Check sheet for the modelled part. Datum: model origin and axes. Units: mm. Face numbers are marked on the shaded views. A direction names the side the tool comes from. Coordinates: 2 decimals unless noted, no trailing zeros. Write each loop counter-clockwise with the first axis right and the second up, starting at its lowest first coordinate (ties: lowest second). Pieces come first, ordered by that corner, then holes. Notation, with made-up numbers: (56, 62) -> (87, 62) arc R21 cw to (87, 71) -> close; hole circle Ø10 at (-21.75, 0.5). An arc over 180 degrees is marked (long way). Put each result on its own line as item: value.
```python
from build123d import *

# Parameters (mm, degrees)
SKETCH1_W           = 8
SKETCH1_H           = 3.056305014
BOSS_EXTRUDE1_DEPTH = 1.5


with BuildPart() as part:
    # Sketch1 → Boss-Extrude1 (new, symmetric)
    with BuildSketch(Plane.XY):
        with BuildLine():
            Line((-10.083709216, 9.599779274), (-10.083709216, 6.299779274))
            Line((-10.083709216, 6.299779274), (-12.68296021, 6.299779274))
            ThreePointArc((-12.68296021, 6.299779274), (-13.0365136, 6.153332664), (-13.18296021, 5.799779274))
            Line((-13.18296021, 5.799779274), (-13.18296021, 4.602368782))
            ThreePointArc((-13.18296021, 4.602368782), (-13.376633784, 4.010897992), (-13.882635601, 3.648531727))
            ThreePointArc((-13.882635601, 3.648531727), (-14.651645992, 3.099880506), (-14.950395595, 2.20369759))
            ThreePointArc((-14.950395595, 2.20369759), (-14.575936583, 1.043545253), (-13.583709216, 0.335267166))
            Line((-13.583709216, 0.335267166), (-13.583709216, 1.664695612))
            Line((-13.583709216, 1.664695612), (-10.083709216, 1.664695612))
            Line((-10.083709216, 1.664695612), (-10.083709216, 0.256084288))
            Line((-10.083709216, 0.256084288), (13.916290784, 0.256084288))
            Line((13.916290784, 0.256084288), (13.916290784, 1.664695612))
            Line((13.916290784, 1.664695612), (17.416290784, 1.664695612))
            Line((17.416290784, 1.664695612), (17.416290784, 0.335267166))
            ThreePointArc((17.416290784, 0.335267166), (18.408518152, 1.043545253), (18.782977164, 2.20369759))
            ThreePointArc((18.782977164, 2.20369759), (18.484227561, 3.099880506), (17.715217169, 3.648531727))
            ThreePointArc((17.715217169, 3.648531727), (17.209215353, 4.010897992), (17.015541778, 4.602368782))
            Line((17.015541778, 4.602368782), (17.015541778, 5.799779274))
            ThreePointArc((17.015541778, 5.799779274), (16.869095169, 6.153332664), (16.515541778, 6.299779274))
            Line((16.515541778, 6.299779274), (13.916290784, 6.299779274))
            Line((13.916290784, 6.299779274), (13.916290784, 9.599779274))
            Line((13.916290784, 9.599779274), (-10.083709216, 9.599779274))
        make_face()
        with Locations((1.916290784, 4.927931781)):
            Rectangle(SKETCH1_W, SKETCH1_H, mode=Mode.SUBTRACT)
    extrude(amount=BOSS_EXTRUDE1_DEPTH, both=True)


solid = part.part
```
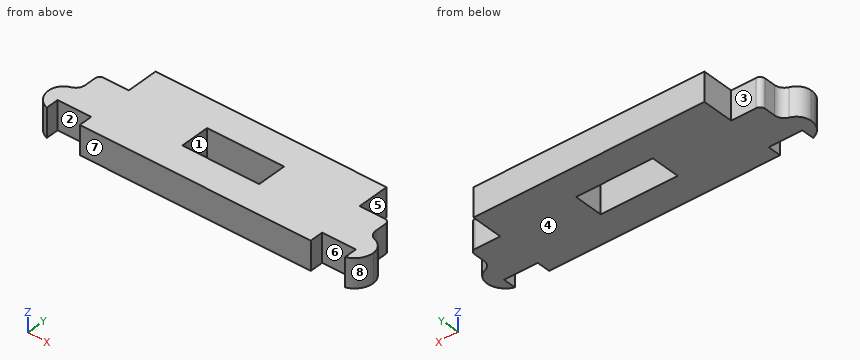
Q1. Mould release check, pull along X, two halves, no side actions. Record for the marked faces 6, 7 and 8: released by +X, released by -X, zero draft, split by the parting line, or undercut.
Recorded:
face 6: undercut
face 7: zero draft
face 8: released by +X
Q2. Tool access check on the marked faces 1, 2, 3, 4 and 5. Record the directions out of +Z, -Z, +X, -X, +Y, -Y that give a thin tool (end or side, any length) a straight path to the whole face; none if there is none.
Recorded:
face 1: +Z, -Z
face 2: +Z, -Z, -Y
face 3: +Z, -Z, -X, +Y
face 4: -Z, +X, -X, +Y, -Y
face 5: +Z, -Z, +X, +Y
Q3. Cross-section at D-D (y = 1). Record the cut outline in (x, z).
Recorded:
outline: (-14.54, -1.5) -> (-13.58, -1.5) -> (-13.58, 1.5) -> (-14.54, 1.5) -> close; (-10.08, -1.5) -> (13.92, -1.5) -> (13.92, 1.5) -> (-10.08, 1.5) -> close; (17.42, -1.5) -> (18.38, -1.5) -> (18.38, 1.5) -> (17.42, 1.5) -> close
Q4. Depth check by flat-ended pin: P1, Ø0.9, axis at x = 15.5, z = -0.5, coming from the -Y side; P2, Ø4, axis at x = 1.5, y = 4, coming from the +Z side; P3, Ø0.6, axis at y = 5, z = 0.5, coming from the -X side; P4, Ø0.7, axis at y = 1, z = 0.5, coming from the -X side. Enter the tip coordinate at first touch or a pass-through.
Recorded:
P1: stops at y = 1.66
P2: stops at z = 1.5
P3: stops at x = -13.18
P4: stops at x = -14.76
Q5. Cross-section at A-A (z = 0.8). Record the cut outline in (x, y).
Recorded:
outline: (-14.95, 2.2) arc R1.94 ccw to (-13.58, 0.34) -> (-13.58, 1.66) -> (-10.08, 1.66) -> (-10.08, 0.26) -> (13.92, 0.26) -> (13.92, 1.66) -> (17.42, 1.66) -> (17.42, 0.34) arc R1.94 ccw to (18.78, 2.2) arc R1.53 ccw to (17.72, 3.65) arc R1 cw to (17.02, 4.6) -> (17.02, 5.8) arc R0.5 ccw to (16.52, 6.3) -> (13.92, 6.3) -> (13.92, 9.6) -> (-10.08, 9.6) -> (-10.08, 6.3) -> (-12.68, 6.3) arc R0.5 ccw to (-13.18, 5.8) -> (-13.18, 4.6) arc R1 cw to (-13.88, 3.65) arc R1.53 ccw to start; hole (-2.08, 3.4) -> (5.92, 3.4) -> (5.92, 6.46) -> (-2.08, 6.46) -> close
Q6. Material ranges on line 1 along Y through (x, z) = (1, -0.5); line 2 along X through (y, z) = (5, 0.05); line 3 along X through (y, z) = (7.5, -1), recorded low to high.
Recorded:
line 1: y = 0.26 to 3.4, 6.46 to 9.6
line 2: x = -13.18 to -2.08, 5.92 to 17.02
line 3: x = -10.08 to 13.92
Q7. Cross-section at C-C (x = -0.5). Record the cut outline in (y, z), plus the area to 3 significant figures.
Recorded:
outline: (0.26, -1.5) -> (3.4, -1.5) -> (3.4, 1.5) -> (0.26, 1.5) -> close; (6.46, -1.5) -> (9.6, -1.5) -> (9.6, 1.5) -> (6.46, 1.5) -> close
area: 18.9 mm2
Q8. Cross-section at B-B (y = 5). Record the cut outline in (x, z), plus the area to 3 significant figures.
Recorded:
outline: (-13.18, -1.5) -> (-2.08, -1.5) -> (-2.08, 1.5) -> (-13.18, 1.5) -> close; (5.92, -1.5) -> (17.02, -1.5) -> (17.02, 1.5) -> (5.92, 1.5) -> close
area: 66.6 mm2
